from build123d import *

# Parameters (mm, degrees)
SKETCH_1_W          = 30
SKETCH_1_H          = 15
EXTRUDE_1_DEPTH     = 4
SKETCH_2_W          = 4
SKETCH_2_H          = 15
EXTRUDE_2_DEPTH     = 15
SKETCH_3_R          = 2
CUT_EXTRUDE_1_DEPTH = 15
SKETCH_4_R          = 3
CUT_EXTRUDE_2_DEPTH = 15


with BuildPart() as part:
    # Эскиз1 → Бобышка-Вытянуть1 (new body)
    with BuildSketch(Plane(origin=(0, 0, 0), x_dir=(1, 0, 0), z_dir=(0, 1, 0))):
        with Locations((15, 7.5)):
            Rectangle(SKETCH_1_W, SKETCH_1_H)
    extrude(amount=EXTRUDE_1_DEPTH)

    # Эскиз2 → Бобышка-Вытянуть2 (add)
    with BuildSketch(Plane(origin=(0, 4, 0), x_dir=(1, 0, 0), z_dir=(0, 1, 0))):
        with Locations((11, 7.5)):
            Rectangle(SKETCH_2_W, SKETCH_2_H)
        with Locations((19, 7.5)):
            Rectangle(SKETCH_2_W, SKETCH_2_H)
    extrude(amount=EXTRUDE_2_DEPTH)

    # Эскиз3 → Вырез-Вытянуть1 (cut)
    with BuildSketch(Plane.XZ):
        with Locations(Location((6, -7.5, 0), (0, 0, 270))):
            Circle(SKETCH_3_R)
        with Locations(Location((24, -7.5, 0), (0, 0, 270))):
            Circle(SKETCH_3_R)
    extrude(amount=-CUT_EXTRUDE_1_DEPTH, mode=Mode.SUBTRACT)

    # Эскиз4 → Вырез-Вытянуть2 (cut)
    with BuildSketch(Plane.ZY.offset(-9)):
        with Locations((-7.5, 13)):
            Circle(SKETCH_4_R)
    extrude(amount=-CUT_EXTRUDE_2_DEPTH, mode=Mode.SUBTRACT)


solid = part.part
Geometry: final body of the model. Coordinates: model frame, mm. A direction names the side the tool comes from. Coordinates: 2 decimals unless noted, no trailing zeros. Loops run counter-clockwise (first coordinate to the right, second up) from the corner with the lowest first, then second, coordinate; pieces in that order, holes last. Notation, with made-up numbers: M 24.5,-24 L 61.5,-24 A31 ccw 61.5,13 Z; hole C 85.5,42.25 d5. An arc over 180 degrees is marked long. One line per item, written item: value. Start each with the question number.
1) Material intervals for L1, parallel to X at y = 1.95, z = -7.5; L2, parallel to Y at x = 18.05, z = -7.5; L3, parallel to X at y = 6.75, z = -4.5, sorted ascending. Write a range as from..to.
2) Pin query (flat end, axial travel): P1, Ø4, axis at y = 10.5, z = -10, coming from the +X side; P2, Ø6, axis at x = 5.5, z = -5, coming from the +Y side; P3, Ø4.5, axis at y = 9, z = -6.5, coming from the -X side; P4, Ø3.5, axis at x = 6, z = -7.5, coming from the +Y side. Return the tip coordinate at first contact, or that it passes through.
3) Reachability of faces 1 (the flat face through (13, 9.7, -7.4)), 2 (the flat face through (21, 9.7, -7.4)), 3 (the flat face through (9, 9.7, -7.4)) from +Z, -Z, +X, -X, +Y, -Y: full face, straight path, thin tool, end or side. Return the list, or none.
4) Draft query along Y for faces 4 (the cylindrical face through (10.97, 11.85, -4.73)), 5 (the flat face through (11, 19, -8)), 6 (the flat face through (15, 0, -8)), 7 (the flat face through (17, 9.7, -7.4)). Return one class per face: released by +Y, released by -Y, zero draft, split by the parting line, or undercut.
5) Cut plane D-D (y = 13). Return loops of the section in (x, z).
6) Cut plane B-B (y = 4.75). Return loops of the section in (x, z), then the cut area to 3 significant figures.
7) Cut plane A-A (x = 6). Return loops of the section in (y, z), then the cut area to 3 significant figures.
8) Cut plane C-C (z = -7.5). Return loops of the section in (x, y).
Evaluation:
1. L1: 0..4, 8..22, 26..30
1. L2: 0..10, 16..19
1. L3: 9..13, 17..21
2. P1: x = 21
2. P2: y = 4
2. P3: x = 9
2. P4: through
3. face 1: +Z, -Z, +Y
3. face 2: +Z, -Z, +X, +Y
3. face 3: +Z, -Z, -X, +Y
4. face 4: undercut
4. face 5: released by +Y
4. face 6: released by -Y
4. face 7: zero draft
5. outline: M 9,-15 L 13,-15 L 13,-10.5 L 9,-10.5 Z; M 9,-4.5 L 13,-4.5 L 13,0 L 9,0 Z; M 17,-15 L 21,-15 L 21,-10.5 L 17,-10.5 Z; M 17,-4.5 L 21,-4.5 L 21,0 L 17,0 Z
6. outline: M 9,-15 L 13,-15 L 13,0 L 9,0 Z; M 17,-15 L 21,-15 L 21,0 L 17,0 Z
6. area: 120 mm^2
7. outline: M 0,-15 L 4,-15 L 4,-9.5 L 0,-9.5 Z; M 0,-5.5 L 4,-5.5 L 4,0 L 0,0 Z
7. area: 44.0 mm^2
8. outline: M 0,0 L 4,0 L 4,4 L 0,4 Z; M 8,0 L 22,0 L 22,4 L 21,4 L 21,10 L 17,10 L 17,4 L 13,4 L 13,10 L 9,10 L 9,4 L 8,4 Z; M 9,16 L 13,16 L 13,19 L 9,19 Z; M 17,16 L 21,16 L 21,19 L 17,19 Z; M 26,0 L 30,0 L 30,4 L 26,4 Z
